Here's how the part is built. I have some questions about the finished solid (model axes, mm). Face numbers are marked on the shaded views. A direction names the side the tool comes from. Coordinates: 2 decimals unless noted, no trailing zeros. Loops run counter-clockwise (first coordinate to the right, second up) from the corner with the lowest first, then second, coordinate; pieces in that order, holes last. Notation, with made-up numbers: (61.5, 6) -> (78.5, 6) arc R20 ccw to (78.5, 24) -> close; hole circle Ø2 at (-30, 21.5). An arc over 180 degrees is marked (long way). Answer as a JSON object with one key per item and string values. Group by question number.
Q1. Thinking about a two-plate mould opening in X: for the marked faces 1, 2, 3 and 4, which applies, released by +X, released by -X, zero draft, split by the parting line, or undercut?
Q2. On a 3-axis mill with a long thin cutter (end or side, diameter ignored), from which of +Z, -Z, +X, -X, +Y, -Y can I reach the whole of each face in a straight line? I mean the marked faces 5 and 6. Say none if no direction works.
Q3. I'm going to push flat-ended pins straight in: pin 1 (7.5 mm diameter, centred on x = 2.5, z = 21.25, fed in from -Y); pin 2 (0.8 mm diameter, centred on x = -39, z = 14.5, fed in from +Y); pin 3 (5 mm diameter, centred on x = -22.5, z = -8.75, fed in from +Y); pin 4 (3 mm diameter, centred on y = 11.5, z = 27.25, fed in from -X). Where does each tip first touch, or does it pass through?
Q4. I want a section at C-C on z = 21.25. Write out the boundary of the cut face in (x, y), then the cut area to 4 significant figures.
Q5. I need wall thicknesses on line 1 (X direction, y = 1.1, z = -8.75); line 2 (X direction, y = 8, z = -18.5); line 3 (Y direction, x = -38.95, z = 27.25). Which ranges of each line are inside material? Lowest first, please.
Q6. I want a section at B-B on y = 16. Write out the boundary of the cut face in (x, z).
Q7. I want a section at A-A on z = 5.5. Write out the boundary of the cut face in (x, y).
Q8. I want a section at D-D on x = 2.5. Write out the boundary of the cut face in (y, z).
```python
from build123d import *

# Parameters (mm, degrees)
SKETCH1_W           = 80
SKETCH1_H           = 74.5
BOSS_EXTRUDE1_DEPTH = 1.5
SKETCH2_W           = 1.5
SKETCH2_H           = 74.5
BOSS_EXTRUDE2_DEPTH = 20
SKETCH3_W           = 1.5
SKETCH3_H           = 74.5
BOSS_EXTRUDE3_DEPTH = 38.5
SKETCH4_R           = 1.6
SKETCH4_R_2         = 6.25
SKETCH4_W           = 19
SKETCH4_H           = 27
SKETCH4_W_2         = 12
SKETCH4_H_2         = 20
CUT_EXTRUDE1_DEPTH  = 40
SKETCH5_R           = 1.6
CUT_EXTRUDE2_DEPTH  = 40
SKETCH6_R           = 1.6
CUT_EXTRUDE3_DEPTH  = 40


with BuildPart() as part:
    # Sketch1 → Boss-Extrude1 (new body)
    with BuildSketch(Plane(origin=(0, 0, 0), x_dir=(1, 0, 0), z_dir=(0, 1, 0))):
        Rectangle(SKETCH1_W, SKETCH1_H)
    extrude(amount=BOSS_EXTRUDE1_DEPTH)

    # Sketch2 → Boss-Extrude2 (add)
    with BuildSketch(Plane(origin=(0, 1.5, 0), x_dir=(1, 0, 0), z_dir=(0, 1, 0))):
        with Locations((-39.25, 0)):
            Rectangle(SKETCH2_W, SKETCH2_H)
    extrude(amount=BOSS_EXTRUDE2_DEPTH)

    # Sketch3 → Boss-Extrude3 (add)
    with BuildSketch(Plane(origin=(0, 1.5, 0), x_dir=(1, 0, 0), z_dir=(0, 1, 0))):
        with Locations((39.25, 0)):
            Rectangle(SKETCH3_W, SKETCH3_H)
    extrude(amount=BOSS_EXTRUDE3_DEPTH)

    # Sketch4 → Cut-Extrude1 (cut)
    with BuildSketch(Plane(origin=(0, 1.5, 0), x_dir=(1, 0, 0), z_dir=(0, 1, 0))):
        with Locations(Location((-22.5, 8.75, 0), (0, 0, 270))):
            Circle(SKETCH4_R)
        with Locations(Location((-22.5, -31.25, 0), (0, 0, 270))):
            Circle(SKETCH4_R)
        with Locations(Location((2.5, -21.25, 0), (0, 0, 270))):
            Circle(SKETCH4_R_2)
        with Locations((-22.5, -11.25)):
            Rectangle(SKETCH4_W, SKETCH4_H)
        with Locations((25, -19.75)):
            Rectangle(SKETCH4_W_2, SKETCH4_H_2)
    extrude(amount=-CUT_EXTRUDE1_DEPTH, mode=Mode.SUBTRACT)

    # Sketch5 → Cut-Extrude2 (cut)
    with BuildSketch(Plane.ZY.offset(40)):
        with Locations((27.25, 11.5)):
            Circle(SKETCH5_R)
        with Locations((-27.25, 11.5)):
            Circle(SKETCH5_R)
    extrude(amount=-CUT_EXTRUDE2_DEPTH, mode=Mode.SUBTRACT)

    # Sketch6 → Cut-Extrude3 (cut)
    with BuildSketch(Plane(origin=(40, 0, 0), x_dir=(0, 0, -1), z_dir=(1, 0, 0))):
        with Locations((-27.25, 20)):
            Circle(SKETCH6_R)
        with Locations((27.25, 20)):
            Circle(SKETCH6_R)
    extrude(amount=-CUT_EXTRUDE3_DEPTH, mode=Mode.SUBTRACT)


solid = part.part
```
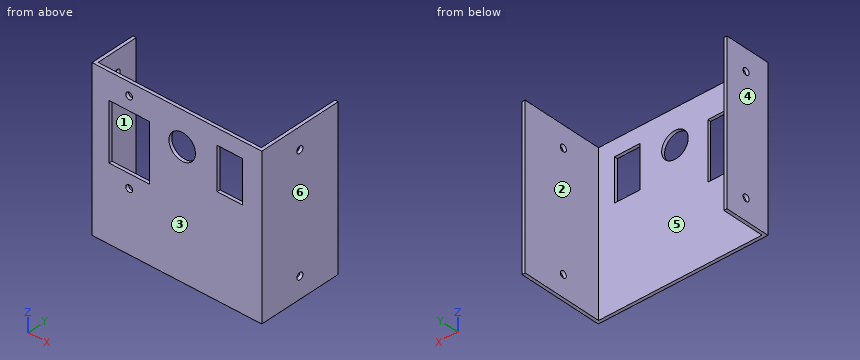
Result set:
{
 "1": {"face 1": "undercut", "face 2": "undercut", "face 3": "zero draft", "face 4": "released by -X"},
 "2": {"face 5": "+Z, -Z, +Y", "face 6": "+Z, -Z, +X, +Y, -Y"},
 "3": {"pin 1": "passes through", "pin 2": "stops at y = 21.5", "pin 3": "stops at y = 1.5", "pin 4": "stops at x = 38.5"},
 "4": {"outline": "(-40, 0) -> (-32, 0) -> (-32, 1.5) -> (-38.5, 1.5) -> (-38.5, 21.5) -> (-40, 21.5) -> close; (-13, 0) -> (-3.75, 0) -> (-3.75, 1.5) -> (-13, 1.5) -> close; (8.75, 0) -> (19, 0) -> (19, 1.5) -> (8.75, 1.5) -> close; (31, 0) -> (40, 0) -> (40, 40) -> (38.5, 40) -> (38.5, 1.5) -> (31, 1.5) -> close", "area": "142.5 mm²"},
 "5": {"line 1": "x = -40 to -24.1, -20.9 to 40", "line 2": "x = -40 to -38.5, 38.5 to 40", "line 3": "y = 0 to 9.9, 13.1 to 21.5"},
 "6": {"outline": "(-40, -37.25) -> (-38.5, -37.25) -> (-38.5, 37.25) -> (-40, 37.25) -> close; (38.5, -37.25) -> (40, -37.25) -> (40, 37.25) -> (38.5, 37.25) -> close"},
 "7": {"outline": "(-40, 0) -> (-32, 0) -> (-32, 1.5) -> (-38.5, 1.5) -> (-38.5, 21.5) -> (-40, 21.5) -> close; (-13, 0) -> (40, 0) -> (40, 40) -> (38.5, 40) -> (38.5, 1.5) -> (-13, 1.5) -> close"},
 "8": {"outline": "(0, -37.25) -> (1.5, -37.25) -> (1.5, 15) -> (0, 15) -> close; (0, 27.5) -> (1.5, 27.5) -> (1.5, 37.25) -> (0, 37.25) -> close"}
}
